from build123d import *

# Parameters (mm, degrees)
F1_DEPTH = 10


with BuildPart() as f1:
    # F0 (on Front) → F1 (new body)
    with BuildSketch(Plane.XZ):
        Polygon((30, -10), (30, 0), (30, 10), (40, 10), (40, 20), (10, 20), (10, 15), (0, 15), (-10, 15), (-10, 20), (-40, 20), (-40, 10), (-30, 10), (-30, 0), (-30, -10), (-40, -10), (-40, -20), (-10, -20), (-10, -15), (0, -15), (10, -15), (10, -20), (40, -20), (40, -10), align=None)
        with BuildLine():
            ThreePointArc((0, 5), (3.535534, 3.535534), (5, 0))
            ThreePointArc((5, 0), (3.535534, -3.535534), (0, -5))
            ThreePointArc((0, -5), (-3.535534, -3.535534), (-5, 0))
            ThreePointArc((-5, 0), (-3.535534, 3.535534), (0, 5))
        make_face(mode=Mode.SUBTRACT)
    extrude(amount=F1_DEPTH)


solid = f1.part
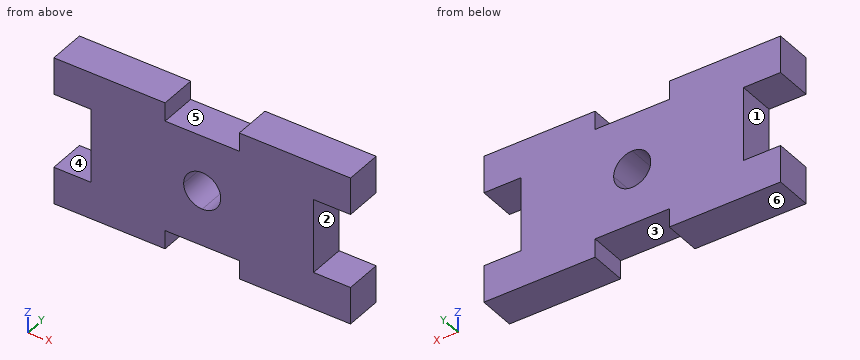
Check sheet for the modelled part. Datum: model origin and axes. Units: mm. Face numbers are marked on the shaded views. A direction names the side the tool comes from. Round coordinates to 2 decimals unless told otherwise and drop trailing zeros. Write each loop counter-clockwise with the first axis right and the second up, starting at its lowest first coordinate (ties: lowest second). Pieces come first, ordered by that corner, then holes. Notation, with made-up numbers: (-12.75, 44.25) - (-6.75, 44.25) arc R21 cw to (-6.75, 49.25) - close; hole circle Ø5 at (38, 8.25). An arc over 180 degrees is marked (long way). Return JSON: item names as keys, results as strings.
Q1. Cross-section at B-B (y = -4). Record the boundary of the cut face in (x, z).
Returned:
{"outline": "(-40, -20) - (-10, -20) - (-10, -15) - (10, -15) - (10, -20) - (40, -20) - (40, -10) - (30, -10) - (30, 10) - (40, 10) - (40, 20) - (10, 20) - (10, 15) - (-10, 15) - (-10, 20) - (-40, 20) - (-40, 10) - (-30, 10) - (-30, -10) - (-40, -10) - close; hole circle Ø10 at (0, 0)"}
Q2. Scan lines: L1, parallel to Z at x = 33, y = -0.5; L2, parallel to X at y = -7.25, z = 17.5; L3, parallel to Z at x = 0.5, y = -2.25. Record each from-to range of solid material in increasing order. Write a range as from..to.
Returned:
{"L1": "z = -20..-10, 10..20", "L2": "x = -40..-10, 10..40", "L3": "z = -15..-4.97, 4.97..15"}
Q3. Access from +Z, -Z, +X, -X, +Y, -Y to the whole of each face (thin tool, end or side, straight path). Record for the marked faces 1, 2 and 3.
Returned:
{"face 1": "-X, +Y, -Y", "face 2": "+X, +Y, -Y", "face 3": "-Z, +Y, -Y"}
Q4. Cross-section at D-D (x = 9). Record the boundary of the cut face in (y, z).
Returned:
{"outline": "(-10, -15) - (0, -15) - (0, 15) - (-10, 15) - close"}
Q5. Depth check by flat-ended pin: P1, Ø4, axis at y = -7, z = 4, coming from the -X side; P2, Ø4, axis at x = 1.5, y = -3, coming from the -Z side; P3, Ø2, axis at y = -4, z = 4, coming from the +X side. Enter the tip coordinate at first touch or a pass-through.
Returned:
{"P1": "stops at x = -30", "P2": "stops at z = -15", "P3": "stops at x = 30"}
Q6. Draft check along Z on the marked faces 4, 5 and 6. Enter one of: released by +Z, released by -Z, zero draft, split by the parting line, or undercut.
Returned:
{"face 4": "undercut", "face 5": "released by +Z", "face 6": "released by -Z"}
Q7. Cross-section at C-C (z = 3.5). Record the boundary of the cut face in (x, y).
Returned:
{"outline": "(-30, -10) - (-3.57, -10) - (-3.57, 0) - (-30, 0) - close; (3.57, -10) - (30, -10) - (30, 0) - (3.57, 0) - close"}
Q8. Cross-section at A-A (x = -34). Record the boundary of the cut face in (y, z).
Returned:
{"outline": "(-10, -20) - (0, -20) - (0, -10) - (-10, -10) - close; (-10, 10) - (0, 10) - (0, 20) - (-10, 20) - close"}
